The listing builds one solid part. Answer for the finished solid, in the listing's coordinates (mm). A direction names the side the tool comes from. Coordinates: 2 decimals unless noted, no trailing zeros. Order: outer loops, then holes, each group sorted by start corner. A loop starts at its lowest first (then second) coordinate and runs counter-clockwise, first axis right, second up. Notation, with made-up numbers: (62, 45.5) -> (103, 45.5) arc R15 ccw to (103, 61.5) -> close; hole circle Ø6 at (3, 60). An arc over 180 degrees is marked (long way). Return JSON: item names as keys, results as strings.
from build123d import *

# Parameters (mm, degrees)
SKETCH1_W           = 95
SKETCH1_H           = 95
BOSS_EXTRUDE1_DEPTH = 50
CUT_EXTRUDE1_DEPTH  = 100
SKETCH3_R           = 9.5
CUT_EXTRUDE2_DEPTH  = 45
CUT_EXTRUDE4_DEPTH  = 45
CUT_EXTRUDE5_DEPTH  = 45
CUT_EXTRUDE6_DEPTH  = 45
CUT_EXTRUDE7_DEPTH  = 45
SKETCH9_R           = 9.5
CUT_EXTRUDE9_DEPTH  = 45
SKETCH11_R          = 9.5
CUT_EXTRUDE10_DEPTH = 45
SKETCH12_W          = 31.985759797
SKETCH12_H          = 95
BOSS_EXTRUDE2_DEPTH = 45
CUT_EXTRUDE11_DEPTH = 100
SKETCH14_R          = 9.5
CUT_EXTRUDE12_DEPTH = 100
SKETCH15_R          = 9.5
CUT_EXTRUDE13_DEPTH = 100
SKETCH16_R          = 9.5
CUT_EXTRUDE14_DEPTH = 100
FILLET2_R           = 4
SKETCH17_W          = 34
SKETCH17_H          = 34
CUT_EXTRUDE16_DEPTH = 22
SKETCH19_W          = 34
SKETCH19_H          = 34
CUT_EXTRUDE17_DEPTH = 22
SKETCH20_W          = 12.5
SKETCH20_H          = 16.5
CUT_EXTRUDE18_DEPTH = 60
CUT_EXTRUDE19_DEPTH = 60
SKETCH22_W          = 99.816433395
SKETCH22_H          = 26.367590903
CUT_EXTRUDE21_DEPTH = 100
SKETCH23_R          = 1
CUT_EXTRUDE24_DEPTH = 909
SKETCH25_R          = 1
CUT_EXTRUDE25_DEPTH = 789
SKETCH27_W          = 26.129652456
SKETCH27_H          = 47
CUT_EXTRUDE27_DEPTH = 9
SKETCH28_W          = 2
SKETCH28_H          = 20
CUT_EXTRUDE28_DEPTH = 5
SKETCH29_W          = 99.017305209
SKETCH29_H          = 17.897343585
CUT_EXTRUDE29_DEPTH = 447
CUT_EXTRUDE30_DEPTH = 447
SKETCH31_W          = 26.129652456
SKETCH31_H          = 47
CUT_EXTRUDE31_DEPTH = 447
SKETCH32_W          = 12.716067022
SKETCH32_H          = 47
CUT_EXTRUDE32_DEPTH = 90
BOSS_EXTRUDE4_DEPTH = 9
SKETCH37_W          = 36.129652456
SKETCH37_H          = 47
CUT_EXTRUDE34_DEPTH = 9
SKETCH38_W          = 16
SKETCH38_H          = 58
CUT_EXTRUDE36_DEPTH = 19
SKETCH40_W          = 8.75
SKETCH40_H          = 1.118077743
BOSS_EXTRUDE5_DEPTH = 48
SKETCH41_W          = 47
SKETCH41_H          = 1.118077743
BOSS_EXTRUDE6_DEPTH = 10
SKETCH42_W          = 32.132900769
SKETCH42_H          = 1
BOSS_EXTRUDE7_DEPTH = 22
SKETCH43_W          = 32.132900769
SKETCH43_H          = 1.118077743
BOSS_EXTRUDE8_DEPTH = 22


with BuildPart() as part:
    # Sketch1 → Boss-Extrude1 (new body)
    with BuildSketch(Plane(origin=(0, 0, 0), x_dir=(1, 0, 0), z_dir=(0, 1, 0))):
        with Locations((-8.446550514, 2.043801884)):
            Rectangle(SKETCH1_W, SKETCH1_H)
    extrude(amount=BOSS_EXTRUDE1_DEPTH)

    # Sketch2 → Cut-Extrude1 (cut)
    with BuildSketch(Plane.XY.offset(45.456198116)):
        Polygon((39.053449486, 0), (36.353449486, 50), (39.053449486, 50), align=None)
    extrude(amount=-CUT_EXTRUDE1_DEPTH, mode=Mode.SUBTRACT)

    # Sketch3 → Cut-Extrude2 (cut)
    with BuildSketch(Plane(origin=(38.939900735, 2.10275464, 0), x_dir=(0, 0, -1), z_dir=(0.998545181, 0.05392144, 0))):
        with Locations((2.043801884, 13.394181776)):
            Circle(SKETCH3_R)
    extrude(amount=-CUT_EXTRUDE2_DEPTH, mode=Mode.SUBTRACT)

    # Sketch5 → Cut-Extrude4 (cut)
    with BuildSketch(Plane(origin=(0, 50, 0), x_dir=(1, 0, 0), z_dir=(0, 1, 0))):
        Polygon((39.053449486, 49.543801884), (39.053449486, 29.543801884), (19.053449486, 49.543801884), align=None)
        Polygon((39.053449486, -45.456198116), (39.053449486, -25.456198116), (19.053449486, -45.456198116), align=None)
    extrude(amount=-CUT_EXTRUDE4_DEPTH, mode=Mode.SUBTRACT)

    # Sketch6 → Cut-Extrude5 (cut)
    with BuildSketch(Plane(origin=(0, 50, 0), x_dir=(1, 0, 0), z_dir=(0, 1, 0))):
        Polygon((19.053449486, -45.456198116), (12.925569587, -39.328318218), (6.797689689, -45.456198116), align=None)
        Polygon((19.053449486, 49.543801884), (12.925569587, 43.415921985), (6.797689689, 49.543801884), align=None)
    extrude(amount=-CUT_EXTRUDE5_DEPTH, mode=Mode.SUBTRACT)

    # Sketch7 → Cut-Extrude6 (cut)
    with BuildSketch(Plane(origin=(-13.201374315, 0, 13.201374315), x_dir=(0.707106781, 0, 0.707106781), z_dir=(-0.707106781, 0, 0.707106781))):
        Polygon((45.615209271, 5), (42.915209271, 50), (45.615209271, 50), align=None)
    extrude(amount=-CUT_EXTRUDE6_DEPTH, mode=Mode.SUBTRACT)

    # Sketch8 → Cut-Extrude7 (cut)
    with BuildSketch(Plane(origin=(-15.245176199, 0, -15.245176199), x_dir=(-0.707106781, 0, 0.707106781), z_dir=(-0.707106781, 0, -0.707106781))):
        Polygon((-48.505581614, 5), (-45.805581614, 50), (-48.505581614, 50), align=None)
    extrude(amount=-CUT_EXTRUDE7_DEPTH, mode=Mode.SUBTRACT)

    # Sketch9 → Cut-Extrude9 (cut)
    with BuildSketch(Plane(origin=(34.386964646, 2.917830706, -34.386964646), x_dir=(-0.708373873, 0.059677836, -0.70331004), z_dir=(0.705837415, 0.059892291, -0.705837415))):
        with Locations((14.526974541, 11.311121921)):
            Circle(SKETCH9_R)
    extrude(amount=-CUT_EXTRUDE9_DEPTH, mode=Mode.SUBTRACT)

    # Sketch11 → Cut-Extrude10 (cut)
    with BuildSketch(Plane(origin=(32.350494057, 2.745030447, 32.350494057), x_dir=(0.70331004, 0.059677836, -0.708373873), z_dir=(0.705837415, 0.059892291, 0.705837415))):
        with Locations((-10.17752107, 12.964151979)):
            Circle(SKETCH11_R)
    extrude(amount=-CUT_EXTRUDE10_DEPTH, mode=Mode.SUBTRACT)

    # Sketch12 → Boss-Extrude2 (add)
    with BuildSketch(Plane(origin=(0, 5, 0), x_dir=(1, 0, 0), z_dir=(0, 1, 0))):
        with Locations((22.790569588, 2.043801884)):
            Rectangle(SKETCH12_W, SKETCH12_H)
    extrude(amount=BOSS_EXTRUDE2_DEPTH)

    # Sketch13 → Cut-Extrude11 (cut)
    with BuildSketch(Plane.XY.offset(45.456198116)):
        Polygon((39.053449486, 0), (29.053449486, 3), (19.053449486, 50), (49.745275601, 50), align=None)
    extrude(amount=-CUT_EXTRUDE11_DEPTH, mode=Mode.SUBTRACT)

    # Sketch14 → Cut-Extrude12 (cut)
    with BuildSketch(Plane(origin=(-5.994632406, -0.32371015, 0), x_dir=(0, 0, -1), z_dir=(0.998545181, 0.05392144, 0))):
        with Locations((2.043801884, 13.394181776)):
            Circle(SKETCH14_R)
    extrude(amount=CUT_EXTRUDE12_DEPTH, mode=Mode.SUBTRACT)

    # Sketch15 → Cut-Extrude13 (cut)
    with BuildSketch(Plane(origin=(0.587810371, 0.049877364, 0.587810371), x_dir=(0.70331004, 0.059677836, -0.708373873), z_dir=(0.705837415, 0.059892291, 0.705837415))):
        with Locations((-10.17752107, 12.964151979)):
            Circle(SKETCH15_R)
    extrude(amount=CUT_EXTRUDE13_DEPTH, mode=Mode.SUBTRACT)

    # Sketch16 → Cut-Extrude14 (cut)
    with BuildSketch(Plane(origin=(2.62428096, 0.222677624, -2.62428096), x_dir=(-0.708373873, 0.059677836, -0.70331004), z_dir=(0.705837415, 0.059892291, -0.705837415))):
        with Locations((14.526974541, 11.311121921)):
            Circle(SKETCH16_R)
    extrude(amount=CUT_EXTRUDE14_DEPTH, mode=Mode.SUBTRACT)

    # Fillet2
    fillet2_edges = [part.edges().sort_by_distance(p)[0] for p in [
        (29.053449486, 3, -2.043801884),
    ]]
    fillet(fillet2_edges, radius=FILLET2_R)

    # Sketch17 → Cut-Extrude16 (cut)
    with BuildSketch(Plane.XY.offset(45.456198116)):
        with Locations((-38.946550514, 17)):
            Rectangle(SKETCH17_W, SKETCH17_H)
    extrude(amount=-CUT_EXTRUDE16_DEPTH, mode=Mode.SUBTRACT)

    # Sketch19 → Cut-Extrude17 (cut)
    with BuildSketch(Plane(origin=(0, 0, -49.543801884), x_dir=(-1, 0, 0), z_dir=(0, 0, -1))):
        with Locations((38.946550514, 17)):
            Rectangle(SKETCH19_W, SKETCH19_H)
    extrude(amount=-CUT_EXTRUDE17_DEPTH, mode=Mode.SUBTRACT)

    # Sketch20 → Cut-Extrude18 (cut)
    with BuildSketch(Plane.XY.offset(23.456198116)):
        with Locations((-38.946550514, 12.25)):
            Rectangle(SKETCH20_W, SKETCH20_H)
    extrude(amount=-CUT_EXTRUDE18_DEPTH, mode=Mode.SUBTRACT)

    # Sketch21 → Cut-Extrude19 (cut)
    with BuildSketch(Plane.XY.offset(23.456198116)):
        Polygon((-55.946550514, 34), (-48.446550514, 0), (-55.946550514, 0), align=None)
    extrude(amount=-CUT_EXTRUDE19_DEPTH, mode=Mode.SUBTRACT)

    # Sketch22 → Cut-Extrude21 (cut)
    with BuildSketch(Plane.XY.offset(45.456198116)):
        with Locations((-7.85416812, 1.233943624)):
            Rectangle(SKETCH22_W, SKETCH22_H)
    extrude(amount=-CUT_EXTRUDE21_DEPTH, mode=Mode.SUBTRACT)

    # Sketch23 → Cut-Extrude24 (cut)
    with BuildSketch(Plane(origin=(0, 14.417739075, 0), x_dir=(-1, 0, 0), z_dir=(0, -1, 0))):
        with Locations((11.946550514, -35.456198116)):
            Circle(SKETCH23_R)
        with Locations((11.946550514, 39.543801884)):
            Circle(SKETCH23_R)
        with Locations((-16.624143299, -12.956198116)):
            Circle(SKETCH23_R)
        with Locations((-16.624143299, 17.043801884)):
            Circle(SKETCH23_R)
    extrude(amount=-CUT_EXTRUDE24_DEPTH, mode=Mode.SUBTRACT)

    # Sketch25 → Cut-Extrude25 (cut)
    with BuildSketch(Plane(origin=(0, 14.417739075, 0), x_dir=(-1, 0, 0), z_dir=(0, -1, 0))):
        with Locations((48.196550514, -13.456198116)):
            Circle(SKETCH25_R)
        with Locations((48.196550514, 17.543801884)):
            Circle(SKETCH25_R)
    extrude(amount=-CUT_EXTRUDE25_DEPTH, mode=Mode.SUBTRACT)

    # Sketch27 → Cut-Extrude27 (cut)
    with BuildSketch(Plane(origin=(0, 14.417739075, 0), x_dir=(-1, 0, 0), z_dir=(0, -1, 0))):
        with Locations((17.631724286, 2.043801884)):
            Rectangle(SKETCH27_W, SKETCH27_H)
    extrude(amount=-CUT_EXTRUDE27_DEPTH, mode=Mode.SUBTRACT)

    # Sketch28 → Cut-Extrude28 (cut)
    with BuildSketch(Plane(origin=(0, 14.417739075, 0), x_dir=(-1, 0, 0), z_dir=(0, -1, 0))):
        with Locations((31.696550514, 2.043801884)):
            Rectangle(SKETCH28_W, SKETCH28_H)
    extrude(amount=-CUT_EXTRUDE28_DEPTH, mode=Mode.SUBTRACT)

    # Sketch29 → Cut-Extrude29 (cut)
    with BuildSketch(Plane.XY.offset(45.456198116)):
        with Locations((-6.437897909, 42.948671793)):
            Rectangle(SKETCH29_W, SKETCH29_H)
    extrude(amount=-CUT_EXTRUDE29_DEPTH, mode=Mode.SUBTRACT)

    # Sketch30 → Cut-Extrude30 (cut)
    with BuildSketch(Plane.XY.offset(45.456198116)):
        Polygon((24.258594843, 25.535816818), (-54.079451283, 25.535816818), (-55.946550514, 34), (22.457704805, 34), align=None)
    extrude(amount=-CUT_EXTRUDE30_DEPTH, mode=Mode.SUBTRACT)

    # Sketch31 → Cut-Extrude31 (cut)
    with BuildSketch(Plane(origin=(0, 23.417739075, 0), x_dir=(-1, 0, 0), z_dir=(0, -1, 0))):
        with Locations((17.631724286, 2.043801884)):
            Rectangle(SKETCH31_W, SKETCH31_H)
    extrude(amount=-CUT_EXTRUDE31_DEPTH, mode=Mode.SUBTRACT)

    # Sketch32 → Cut-Extrude32 (cut)
    with BuildSketch(Plane(origin=(0, 14.417739075, 0), x_dir=(-1, 0, 0), z_dir=(0, -1, 0))):
        with Locations((0.924931569, 2.043801884)):
            Rectangle(SKETCH32_W, SKETCH32_H)
    extrude(amount=-CUT_EXTRUDE32_DEPTH, mode=Mode.SUBTRACT)

    # Sketch35 → Boss-Extrude4 (add)
    with BuildSketch(Plane(origin=(0, 25.535816818, 0), x_dir=(1, 0, 0), z_dir=(0, 1, 0))):
        Polygon((-54.079451283, 27.543801884), (-21.946550514, 27.543801884), (-21.946550514, 49.543801884), (24.258594843, 49.543801884), (24.258594843, -45.456198116), (-21.946550514, -45.456198116), (-21.946550514, -23.456198116), (-54.079451283, -23.456198116), align=None)
    extrude(amount=BOSS_EXTRUDE4_DEPTH)

    # Sketch37 → Cut-Extrude34 (cut)
    with BuildSketch(Plane(origin=(0, 25.535816818, 0), x_dir=(-1, 0, 0), z_dir=(0, -1, 0))):
        with Locations((12.631724286, 2.043801884)):
            Rectangle(SKETCH37_W, SKETCH37_H)
    extrude(amount=-CUT_EXTRUDE34_DEPTH, mode=Mode.SUBTRACT)

    # Sketch38 → Cut-Extrude36 (cut)
    with BuildSketch(Plane(origin=(0, 14.417739075, 0), x_dir=(-1, 0, 0), z_dir=(0, -1, 0))):
        with Locations((22.696550514, 2.043801884)):
            Rectangle(SKETCH38_W, SKETCH38_H)
    extrude(amount=-CUT_EXTRUDE36_DEPTH, mode=Mode.SUBTRACT)

    # Sketch40 → Boss-Extrude5 (add)
    with BuildSketch(Plane.XY.offset(-25.543801884)):
        with Locations((-26.321550514, 33.976777947)):
            Rectangle(SKETCH40_W, SKETCH40_H)
    extrude(amount=BOSS_EXTRUDE5_DEPTH)

    # Sketch41 → Boss-Extrude6 (add)
    with BuildSketch(Plane(origin=(-21.946550514, 0, 0), x_dir=(0, 0, -1), z_dir=(1, 0, 0))):
        with Locations((2.043801884, 33.976777947)):
            Rectangle(SKETCH41_W, SKETCH41_H)
    extrude(amount=BOSS_EXTRUDE6_DEPTH)

    # Sketch42 → Boss-Extrude7 (add)
    with BuildSketch(Plane.XY.offset(23.456198116)):
        with Locations((-38.013000899, 34.035816818)):
            Rectangle(SKETCH42_W, SKETCH42_H)
    extrude(amount=BOSS_EXTRUDE7_DEPTH)

    # Sketch43 → Boss-Extrude8 (add)
    with BuildSketch(Plane(origin=(0, 0, -27.543801884), x_dir=(-1, 0, 0), z_dir=(0, 0, -1))):
        with Locations((38.013000899, 33.976777947)):
            Rectangle(SKETCH43_W, SKETCH43_H)
    extrude(amount=BOSS_EXTRUDE8_DEPTH)


solid = part.part
1. The part is cut by section A-A on y = 32.25. Give the vertices of the cut face in (x, z).
Answer block:
{"outline": "(-54.08, -27.54) -> (-30.7, -27.54) -> (-30.7, 23.46) -> (-54.08, 23.46) -> close; (-21.95, -49.54) -> (24.26, -49.54) -> (24.26, 45.46) -> (-21.95, 45.46) -> (-21.95, 26.96) -> (-14.7, 26.96) -> (-14.7, 21.46) -> (5.43, 21.46) -> (5.43, -25.54) -> (-14.7, -25.54) -> (-14.7, -31.04) -> (-21.95, -31.04) -> close"}
2. Consider line 1 (Z direction, x = 1, y = 33.5); line 2 (X direction, y = 21, z = -26); line 3 (Z direction, x = -21, y = 15.5). Determine where each line is inside the solid, lowest interval first. Write a range as from..to.
Answer block:
{"line 1": "z = -49.54..-25.54, 21.46..45.46", "line 2": "x = -53.08..-30.7, -14.7..-1.31, 15.46..25.22", "line 3": "z = -49.54..-31.04, 26.96..45.46"}
3. Determine the mould class of faces 1 (the face through (-39, 20.5, -2)), 2 (the face through (17, 25.536, 13)), 3 (the face through (-43, 26, -27.544)) for opening direction Z: pulls with the +Z half, pulls with the -Z half, needs draft (parallel to the pull), parting line crosses it, or undercut.
Answer block:
{"face 1": "needs draft", "face 2": "undercut", "face 3": "pulls with the -Z half"}
4. The part is cut by section B-B on x = -16.5. Give the vertices of the cut face in (y, z).
Answer block:
{"outline": "(14.42, -49.54) -> (34.54, -49.54) -> (34.54, 45.46) -> (14.42, 45.46) -> (14.42, 26.96) -> (33.42, 26.96) -> (33.42, -31.04) -> (14.42, -31.04) -> close"}
5. Each of these flat-tipped pins is pushed along its axis until it touches: pin 1 Ø1 at (x, z) = (-32, -6) entering from -Y; pin 2 Ø0.6 at (x, z) = (16.5, 13) entering from -Y; pin 3 Ø2 at (x, y) = (-32, 17) entering from -Z. Where does it stop, or does it pass through?
Answer block:
{"pin 1": "stops at y = 19.42", "pin 2": "stops at y = 25.54", "pin 3": "stops at z = -27.54"}
6. For faces 4 (the face through (-45.197, 17, -2)), 5 (the face through (-48.658, 19.899, -16.657)), 6 (the face through (-52.87, 20.05, -1.69)), determine the directions among +Z, -Z, +X, -X, +Y, -Y from which every point of the face is accessible in a straight line to the end or side of a thin tool.
Answer block:
{"face 4": "+Z, -Z, -Y", "face 5": "-Y", "face 6": "+Z, -Z, -X, -Y"}
7. The part is cut by section C-C on x = -42. Give the vertices of the cut face in (y, z).
Answer block:
{"outline": "(20.5, -27.54) -> (33.42, -27.54) -> (33.42, -49.54) -> (34.54, -49.54) -> (34.54, 45.46) -> (33.54, 45.46) -> (33.54, 23.46) -> (20.5, 23.46) -> close"}
